```python
from build123d import *

# Parameters (mm, degrees)
SKETCH1_R           = 1.4
BOSS_EXTRUDE3_DEPTH = 6.5
BOSS_EXTRUDE4_DEPTH = 1
CHAMFER1_SIZE       = 0.25
SKETCH4_W           = 2.4
SKETCH4_H           = 0.8
CUT_EXTRUDE1_DEPTH  = 3.6


with BuildPart() as part:
    # Sketch1 → Boss-Extrude3 (new body)
    with BuildSketch(Plane(origin=(0, 0, 0), x_dir=(1, 0, 0), z_dir=(0, 1, 0))):
        with Locations(Location((0, 0, 0), (0, 0, 90))):
            Circle(SKETCH1_R)
    extrude(amount=BOSS_EXTRUDE3_DEPTH)

    # Sketch3 → Boss-Extrude4 (add)
    with BuildSketch(Plane(origin=(0, 0, 0), x_dir=(1, 0, 0), z_dir=(0, 1, 0))):
        with BuildLine():
            Line((-1.4, 0), (-1.4, -1.949358869))
            ThreePointArc((-1.4, -1.949358869), (0, -2.4), (1.4, -1.949358869))
            Line((1.4, -1.949358869), (1.4, 0))
            ThreePointArc((1.4, 0), (0, -1.4), (-1.4, 0))
        make_face()
        with BuildLine():
            Line((-1.4, 1.949358869), (-1.4, 0))
            ThreePointArc((-1.4, 0), (0, 1.4), (1.4, 0))
            Line((1.4, 0), (1.4, 1.949358869))
            ThreePointArc((1.4, 1.949358869), (0, 2.4), (-1.4, 1.949358869))
        make_face()
    extrude(amount=BOSS_EXTRUDE4_DEPTH)

    # Chamfer1
    chamfer1_edges = [part.edges().sort_by_distance(p)[0] for p in [
        (0, 6.5, 1.4),
    ]]
    chamfer(chamfer1_edges, length=CHAMFER1_SIZE)

    # Sketch4 → Cut-Extrude1 (cut)
    with BuildSketch(Plane(origin=(1.4, 0, 0), x_dir=(0, 0, -1), z_dir=(1, 0, 0))):
        Rectangle(SKETCH4_W, SKETCH4_H)
    extrude(amount=-CUT_EXTRUDE1_DEPTH, mode=Mode.SUBTRACT)


solid = part.part
```
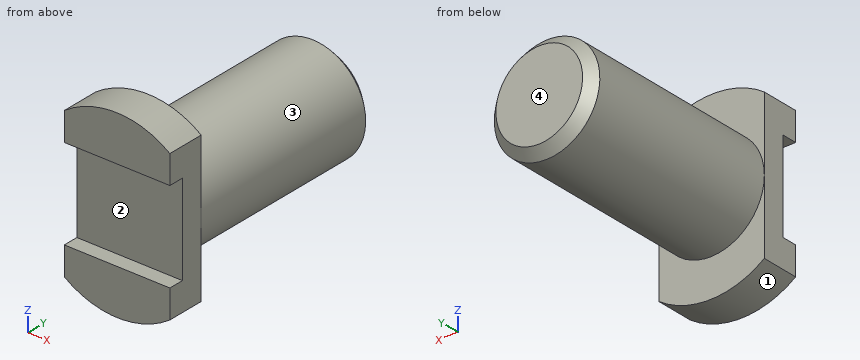
The model under review builds one solid part; all positions refer to its coordinate system, in mm. Face numbers are marked on the shaded views. Round coordinates to 2 decimals unless told otherwise and drop trailing zeros. Order: outer loops, then holes, each group sorted by start corner. A loop starts at its lowest first (then second) coordinate and runs counter-clockwise, first axis right, second up. Notation, with made-up numbers: (47.5, 65) -> (95.5, 65) arc R25 cw to (95.5, 87) -> close; hole circle Ø2 at (80, 46). An arc over 180 degrees is marked (long way). One line per item, written item: value. Start each with the question number.
Q1. Take a section at A-A (x = 0). Write out the cut boundary in (y, z), and give its area (3 significant figures).
Q2. Mouldability with a two-part tool opening along Z and no side actions: class the marked faces 1, 2, 3 and 4 as released by +Z, released by -Z, zero draft, split by the parting line, or undercut.
Q3. Take a section at C-C (y = 2). Write out the cut boundary in (x, z).
Q4. Take a section at B-B (z = -1.65). Write out the cut boundary in (x, y).
Q5. Wall thickness on line 1 (Y direction, x = 0.45, z = 0.75); line 2 (Y direction, x = 0.25, z = 2); line 3 (Z direction, x = -1.1, y = 2.25): over which ranges is each line inside the solid? List them lowest first.
Reported:
1. outline: (0, -2.4) -> (1, -2.4) -> (1, -1.4) -> (6.25, -1.4) -> (6.5, -1.15) -> (6.5, 1.15) -> (6.25, 1.4) -> (1, 1.4) -> (1, 2.4) -> (0, 2.4) -> (0, 1.2) -> (0.4, 1.2) -> (0.4, -1.2) -> (0, -1.2) -> close
1. area: 19.2 mm2
2. face 1: released by -Z
2. face 2: undercut
2. face 3: split by the parting line
2. face 4: zero draft
3. outline: circle Ø2.8 at (0, 0)
4. outline: (-1.4, 0) -> (1.4, 0) -> (1.4, 1) -> (-1.4, 1) -> close
5. line 1: y = 0.4 to 6.5
5. line 2: y = 0 to 1
5. line 3: z = -0.87 to 0.87
